Check sheet for the modelled part. Datum: model origin and axes. Units: mm. Give positions to 0.01 mm unless a question says otherwise; leave off trailing zeros. Use one line per item in the form item = value.
from build123d import *

# Parameters (mm, degrees)
BOSS_EXTRUDE1_DEPTH = 6.35


with BuildPart() as part:
    # Imported Profile → Boss-Extrude1 (new body)
    with BuildSketch(Plane(origin=(0, 0, 0), x_dir=(1, 0, 0), z_dir=(0, 1, 0))):
        with BuildLine():
            add(Edge.make_bspline(
                [(47.6487744, 3.4752534), (40.59301, 8.6201504), (33.5374742, 13.7602468), (26.4818876, 18.9072012)],
                knots=[0, 0, 0, 0, 1, 1, 1, 1], degree=3))
            add(Edge.make_bspline(
                [(26.4818876, 18.9072012), (22.9609904, 21.4772494), (19.4332098, 24.0472976), (15.9054292, 26.6173458)],
                knots=[0, 0, 0, 0, 1, 1, 1, 1], degree=3))
            add(Edge.make_bspline(
                [(15.9054292, 26.6173458), (12.3776486, 29.194252), (8.8292178, 31.722949), (5.3289962, 34.3343484)],
                knots=[0, 0, 0, 0, 1, 1, 1, 1], degree=3))
            add(Edge.make_bspline(
                [(5.3289962, 34.3343484), (1.725422, 37.0214906), (-0.1831594, 41.396793), (0.2922778, 45.8616304)],
                knots=[0, 0, 0, 0, 1, 1, 1, 1], degree=3))
            add(Edge.make_bspline(
                [(0.2922778, 45.8616304), (0.5678678, 48.4454454), (1.3533628, 49.775237), (2.4489156, 52.0214352)],
                knots=[0, 0, 0, 0, 1, 1, 1, 1], degree=3))
            add(Edge.make_bspline(
                [(2.4489156, 52.0214352), (3.406648, 53.9851346), (4.3712638, 55.9420014), (5.3289962, 57.898792)],
                knots=[0, 0, 0, 0, 1, 1, 1, 1], degree=3))
            add(Edge.make_bspline(
                [(5.3289962, 57.898792), (9.1599258, 65.7398482), (12.9977896, 73.5809044), (16.8287192, 81.4287932)],
                knots=[0, 0, 0, 0, 1, 1, 1, 1], degree=3))
            add(Edge.make_bspline(
                [(16.8287192, 81.4287932), (17.2627798, 82.3038486), (19.17827, 86.3001322), (19.7019418, 87.1338872)],
                knots=[0, 0, 0, 0, 1, 1, 1, 1], degree=3))
            add(Edge.make_bspline(
                [(19.7019418, 87.1338872), (20.9490564, 89.1182368), (22.464903, 90.5238474), (24.531955, 91.6194002)],
                knots=[0, 0, 0, 0, 1, 1, 1, 1], degree=3))
            add(Edge.make_bspline(
                [(24.531955, 91.6194002), (26.6885928, 92.7563042), (28.769437, 93.2041316), (31.2085736, 93.0594532)],
                knots=[0, 0, 0, 0, 1, 1, 1, 1], degree=3))
            add(Edge.make_bspline(
                [(31.2085736, 93.0594532), (33.8061554, 92.9079422), (34.9912686, 92.2394904), (37.2925594, 91.2472902)],
                knots=[0, 0, 0, 0, 1, 1, 1, 1], degree=3))
            add(Edge.make_bspline(
                [(37.2925594, 91.2472902), (45.3403208, 87.7540028), (53.505227, 85.3975432), (62.179962, 84.0608428)],
                knots=[0, 0, 0, 0, 1, 1, 1, 1], degree=3))
            add(Edge.make_bspline(
                [(62.179962, 84.0608428), (71.9502752, 82.5518796), (78.5372572, 82.8688462), (88.3282714, 82.8688462)],
                knots=[0, 0, 0, 0, 1, 1, 1, 1], degree=3))
            add(Edge.make_bspline(
                [(88.3282714, 82.8688462), (97.0650078, 82.8688462), (105.8017696, 82.8688462), (114.5316734, 82.8688462)],
                knots=[0, 0, 0, 0, 1, 1, 1, 1], degree=3))
            add(Edge.make_bspline(
                [(114.5316734, 82.8688462), (118.8517562, 82.8688462), (123.1719152, 82.8688462), (127.4989576, 82.8688462)],
                knots=[0, 0, 0, 0, 1, 1, 1, 1], degree=3))
            add(Edge.make_bspline(
                [(127.4989576, 82.8688462), (129.648712, 82.8688462), (131.7984664, 82.9378326), (133.941312, 82.8638424)],
                knots=[0, 0, 0, 0, 1, 1, 1, 1], degree=3))
            add(Edge.make_bspline(
                [(133.941312, 82.8638424), (136.2426282, 82.7813432), (138.1925608, 82.1885834), (140.1493768, 80.9758858)],
                knots=[0, 0, 0, 0, 1, 1, 1, 1], degree=3))
            add(Edge.make_bspline(
                [(140.1493768, 80.9758858), (142.2439624, 79.6874454), (143.6978076, 78.1095974), (144.8071272, 75.9116338)],
                knots=[0, 0, 0, 0, 1, 1, 1, 1], degree=3))
            add(Edge.make_bspline(
                [(144.8071272, 75.9116338), (145.8337698, 73.892791), (146.17827, 71.8946492), (146.17827, 69.669152)],
                knots=[0, 0, 0, 0, 1, 1, 1, 1], degree=3))
            add(Edge.make_bspline(
                [(146.17827, 69.669152), (146.17827, 65.3489422), (146.17827, 61.0219506), (146.17827, 56.7017408)],
                knots=[0, 0, 0, 0, 1, 1, 1, 1], degree=3))
            add(Edge.make_bspline(
                [(146.17827, 56.7017408), (146.17827, 52.3953994), (146.17827, 48.0890326), (146.17827, 43.7826912)],
                knots=[0, 0, 0, 0, 1, 1, 1, 1], degree=3))
            add(Edge.make_bspline(
                [(146.17827, 43.7826912), (146.17827, 41.653587), (146.2542668, 39.586535), (145.5788046, 37.4850406)],
                knots=[0, 0, 0, 0, 1, 1, 1, 1], degree=3))
            add(Edge.make_bspline(
                [(145.5788046, 37.4850406), (144.8415696, 35.176841), (143.6909242, 33.4060546), (141.8650198, 31.8006476)],
                knots=[0, 0, 0, 0, 1, 1, 1, 1], degree=3))
            add(Edge.make_bspline(
                [(141.8650198, 31.8006476), (140.0804666, 30.2296322), (138.2063276, 29.313251), (135.8636602, 28.8653982)],
                knots=[0, 0, 0, 0, 1, 1, 1, 1], degree=3))
            add(Edge.make_bspline(
                [(135.8636602, 28.8653982), (134.2513698, 28.5624016), (131.137025, 28.6449008), (129.5247092, 28.6449008)],
                knots=[0, 0, 0, 0, 1, 1, 1, 1], degree=3))
            add(Edge.make_bspline(
                [(129.5247092, 28.6449008), (127.3818128, 28.6449008), (125.2321092, 28.5624016), (123.0892636, 28.6449008)],
                knots=[0, 0, 0, 0, 1, 1, 1, 1], degree=3))
            add(Edge.make_bspline(
                [(123.0892636, 28.6449008), (120.787922, 28.734385), (118.7139612, 30.0573948), (117.6735772, 32.11068)],
                knots=[0, 0, 0, 0, 1, 1, 1, 1], degree=3))
            add(Edge.make_bspline(
                [(117.6735772, 32.11068), (116.5849078, 34.23285), (117.0741118, 36.3136942), (116.9707592, 38.4427476)],
                knots=[0, 0, 0, 0, 1, 1, 1, 1], degree=3))
            add(Edge.make_bspline(
                [(116.9707592, 38.4427476), (116.8537668, 40.750998), (115.5031726, 42.8042324), (113.4292118, 43.8239916)],
                knots=[0, 0, 0, 0, 1, 1, 1, 1], degree=3))
            add(Edge.make_bspline(
                [(113.4292118, 43.8239916), (111.4448114, 44.8023996), (109.1021694, 44.671488), (107.2349138, 43.4934868)],
                knots=[0, 0, 0, 0, 1, 1, 1, 1], degree=3))
            add(Edge.make_bspline(
                [(107.2349138, 43.4934868), (105.188512, 42.1981376), (104.2790142, 40.1655026), (104.2790142, 37.8228352)],
                knots=[0, 0, 0, 0, 1, 1, 1, 1], degree=3))
            add(Edge.make_bspline(
                [(104.2790142, 37.8228352), (104.2790142, 33.509585), (104.2790142, 29.1963348), (104.2790142, 24.8762012)],
                knots=[0, 0, 0, 0, 1, 1, 1, 1], degree=3))
            add(Edge.make_bspline(
                [(104.2790142, 24.8762012), (104.2790142, 23.7806484), (104.2240232, 22.747097), (103.7900134, 21.6998042)],
                knots=[0, 0, 0, 0, 1, 1, 1, 1], degree=3))
            add(Edge.make_bspline(
                [(103.7900134, 21.6998042), (103.3350232, 20.6180436), (102.7013694, 19.7980808), (101.7643126, 19.0884302)],
                knots=[0, 0, 0, 0, 1, 1, 1, 1], degree=3))
            add(Edge.make_bspline(
                [(101.7643126, 19.0884302), (100.8823738, 18.42008), (99.8833156, 18.0617876), (98.9048568, 17.6207928)],
                knots=[0, 0, 0, 0, 1, 1, 1, 1], degree=3))
            add(Edge.make_bspline(
                [(98.9048568, 17.6207928), (97.9264742, 17.1727876), (96.9480662, 16.7250872), (95.9627748, 16.2772344)],
                knots=[0, 0, 0, 0, 1, 1, 1, 1], degree=3))
            add(Edge.make_bspline(
                [(95.9627748, 16.2772344), (88.0459758, 12.6667514), (80.129126, 9.0562938), (72.2053674, 5.4458362)],
                knots=[0, 0, 0, 0, 1, 1, 1, 1], degree=3))
            add(Edge.make_bspline(
                [(72.2053674, 5.4458362), (70.2279266, 4.5501306), (68.2504096, 3.6474908), (66.272918, 2.7449018)],
                knots=[0, 0, 0, 0, 1, 1, 1, 1], degree=3))
            add(Edge.make_bspline(
                [(66.272918, 2.7449018), (64.2954772, 1.8422874), (62.3868704, 0.8983472), (60.2026736, 0.4917948)],
                knots=[0, 0, 0, 0, 1, 1, 1, 1], degree=3))
            add(Edge.make_bspline(
                [(60.2026736, 0.4917948), (55.779162, -0.3350006), (51.2247642, 0.7467854), (47.6487744, 3.4752534)],
                knots=[0, 0, 0, 0, 1, 1, 1, 1], degree=3))
        make_face()
        with BuildLine():
            add(Edge.make_bspline(
                [(87.8114576, 25.9559044), (87.8114576, 27.7059898), (86.3921056, 29.1253418), (84.6351114, 29.1253418)],
                knots=[0, 0, 0, 0, 1, 1, 1, 1], degree=3))
            add(Edge.make_bspline(
                [(84.6351114, 29.1253418), (82.8781172, 29.1253418), (81.4587144, 27.7059898), (81.4587144, 25.9559044)],
                knots=[0, 0, 0, 0, 1, 1, 1, 1], degree=3))
            add(Edge.make_bspline(
                [(81.4587144, 25.9559044), (81.4587144, 24.198834), (82.8781172, 22.779482), (84.6351114, 22.779482)],
                knots=[0, 0, 0, 0, 1, 1, 1, 1], degree=3))
            add(Edge.make_bspline(
                [(84.6351114, 22.779482), (86.3921056, 22.779482), (87.8114576, 24.198834), (87.8114576, 25.9559044)],
                knots=[0, 0, 0, 0, 1, 1, 1, 1], degree=3))
        make_face(mode=Mode.SUBTRACT)
        with BuildLine():
            add(Edge.make_bspline(
                [(16.5875716, 46.0338932), (15.7469586, 48.059594), (13.4249668, 49.0242352), (11.399266, 48.1836476)],
                knots=[0, 0, 0, 0, 1, 1, 1, 1], degree=3))
            add(Edge.make_bspline(
                [(11.399266, 48.1836476), (9.3735398, 47.3430346), (8.4158074, 45.0210428), (9.249537, 42.9952912)],
                knots=[0, 0, 0, 0, 1, 1, 1, 1], degree=3))
            add(Edge.make_bspline(
                [(9.249537, 42.9952912), (10.0901246, 40.9695904), (12.4121164, 40.0118326), (14.4378172, 40.8455368)],
                knots=[0, 0, 0, 0, 1, 1, 1, 1], degree=3))
            add(Edge.make_bspline(
                [(14.4378172, 40.8455368), (16.4635434, 41.6862006), (17.4212758, 44.0081416), (16.5875716, 46.0338932)],
                knots=[0, 0, 0, 0, 1, 1, 1, 1], degree=3))
        make_face(mode=Mode.SUBTRACT)
        with BuildLine():
            add(Edge.make_bspline(
                [(60.3200216, 18.6384946), (58.9140046, 20.3196952), (56.4128666, 20.5401926), (54.731666, 19.1274954)],
                knots=[0, 0, 0, 0, 1, 1, 1, 1], degree=3))
            add(Edge.make_bspline(
                [(54.731666, 19.1274954), (53.0504654, 17.7218848), (52.829968, 15.2207468), (54.2426652, 13.5395462)],
                knots=[0, 0, 0, 0, 1, 1, 1, 1], degree=3))
            add(Edge.make_bspline(
                [(54.2426652, 13.5395462), (55.6551592, 11.8583456), (58.1563226, 11.6447316), (59.8375232, 13.0505454)],
                knots=[0, 0, 0, 0, 1, 1, 1, 1], degree=3))
            add(Edge.make_bspline(
                [(59.8375232, 13.0505454), (61.511815, 14.4561306), (61.7323124, 16.964152), (60.3200216, 18.6384946)],
                knots=[0, 0, 0, 0, 1, 1, 1, 1], degree=3))
        make_face(mode=Mode.SUBTRACT)
    extrude(amount=BOSS_EXTRUDE1_DEPTH)


solid = part.part
1) Depth check by flat-ended pin: pin 1 Ø2 at (x, y) = (84, 5) entering from -Z; pin 2 Ø2 at (x, z) = (55.5, -58) entering from -Y; pin 3 Ø3 at (x, y) = (20.5, 2) entering from -Z. Enter the tip coordinate at first touch or a pass-through.
Evaluation:
pin_1 = -82.86
pin_2 = 0
pin_3 = -89.88
2) Section check A-A (y = 4.5). State how many separate pieces and enclosed holes the cut face has, then the cut area to 3 significant figures.
Evaluation:
separate_pieces = 1
enclosed_holes = 3
area = 9,020 mm^2
3) Scan lines: line 1 (X direction, y = 6, z = -45); line 2 (Z direction, x = 131, y = 5); line 3 (X direction, y = 2.25, z = -60). Record each from-to range of solid material in increasing order.
Evaluation:
line_1 = 0.23 to 8.98, 16.86 to 146.18
line_2 = -82.9 to -28.64
line_3 = 6.36 to 146.18
